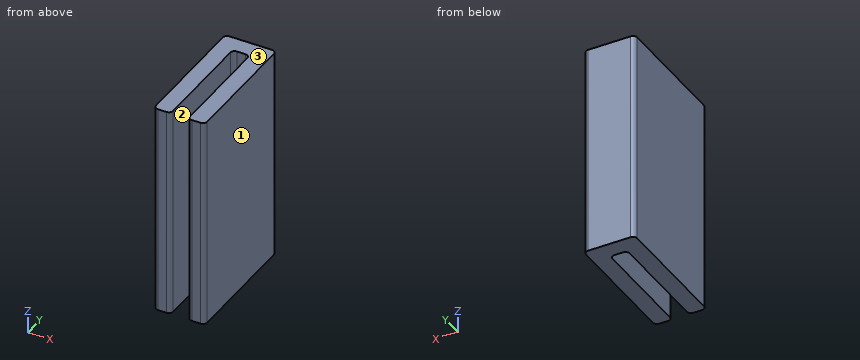
```python
from build123d import *

# Parameters (mm, degrees)
F0_W     = 2
F0_H     = 2
F1_DEPTH = 25
F2_R     = 0.5


with BuildPart() as f1:
    # F0 (on Top) → F1 (new body)
    with BuildSketch(Plane.XY):
        Polygon((2, 0), (0, 0), (0, -15), (2, -15), (2, -2), align=None)
        with Locations((3, -1)):
            Rectangle(F0_W, F0_H)
        Polygon((6, 0), (4, 0), (4, -2), (4, -15), (6, -15), align=None)
    extrude(amount=F1_DEPTH)

    # F2
    f2_edges = [f1.edges().sort_by_distance(p)[0] for p in [
        (2, -2, 12.5),
        (4, -2, 12.5),
        (0, 0, 12.5),
        (6, 0, 12.5),
        (0, -15, 12.5),
        (2, -15, 12.5),
        (4, -15, 12.5),
        (6, -15, 12.5),
    ]]
    fillet(f2_edges, radius=F2_R)


solid = f1.part
```
Geometry check sheet. Reference: the model listing, model coordinates, mm. Face numbers are marked on the shaded views. Give positions to 0.01 mm unless a question says otherwise; leave off trailing zeros. Order: outer loops, then holes, each group sorted by start corner. A loop starts at its lowest first (then second) coordinate and runs counter-clockwise, first axis right, second up. Notation, with made-up numbers: (40.25, 49.25) - (46.25, 49.25) arc R24 ccw to (46.25, 73.25) - close; hole circle Ø1 at (-37.75, -7.5). An arc over 180 degrees is marked (long way). Write item = value, one per line. Start each with the question number.
1) Section check A-A (y = -6.75). Enter the section's corners in (x, z).
2) Scan lines: L1, parallel to X at y = -7.5, z = 9.5; L2, parallel to Y at x = 2.6, z = 9.5; L3, parallel to Y at x = 4.2, z = 10.5. Record each from-to range of solid material in increasing order.
3) Section check B-B (z = 22). Enter the section's corners in (x, y), then the cut area to 3 significant figures.
4) Draft check along X on the marked faces 1, 2 and 3. Enter one of: released by +X, released by -X, zero draft, split by the parting line, or undercut.
5) Gauge pin test, flat end, axial feed: pin 1 Ø1.5 at (x, y) = (1.5, -6.5) entering from -Z. Record the tip position at first contact, or that the pin passes through.
6) Section check C-C (x = 2.8). Enter the section's corners in (y, z).
Geometry check:
q1.outline = (0, 0) - (2, 0) - (2, 25) - (0, 25) - close; (4, 0) - (6, 0) - (6, 25) - (4, 25) - close
q2.L1 = 0 to 2, 4 to 6
q2.L2 = -2 to 0
q2.L3 = -14.9 to 0
q3.outline = (0, -14.5) arc R0.5 ccw to (0.5, -15) - (1.5, -15) arc R0.5 ccw to (2, -14.5) - (2, -2.5) arc R0.5 cw to (2.5, -2) - (3.5, -2) arc R0.5 cw to (4, -2.5) - (4, -14.5) arc R0.5 ccw to (4.5, -15) - (5.5, -15) arc R0.5 ccw to (6, -14.5) - (6, -0.5) arc R0.5 ccw to (5.5, 0) - (0.5, 0) arc R0.5 ccw to (0, -0.5) - close
q3.area = 63.8 mm2
q4.face_1 = released by +X
q4.face_2 = undercut
q4.face_3 = zero draft
q5.pin_1 = 0
q6.outline = (-2, 0) - (0, 0) - (0, 25) - (-2, 25) - close
